Read the model definition and answer for the solid it produces. Units are mm, in the model's axes. Face numbers are marked on the shaded views. A direction names the side the tool comes from. Give positions to 0.01 mm unless a question says otherwise; leave off trailing zeros. Write each loop counter-clockwise with the first axis right and the second up, starting at its lowest first coordinate (ties: lowest second). Pieces come first, ordered by that corner, then holes. Notation, with made-up numbers: (-11.75, 57) -> (27.25, 57) arc R24 cw to (27.25, 78) -> close; hole circle Ø9 at (34.5, -11.5). An arc over 180 degrees is marked (long way). Answer as CSV lines item,"result". Start each with the question number.
1. Given pin 1 (1 mm diameter, centred on y = 27, z = 1, fed in from +X); pin 2 (19.5 mm diameter, centred on x = -9.5, z = -12.5, fed in from +Y); pin 3 (4.5 mm diameter, centred on x = -7.75, y = 12.78, fed in from -Z), each flat-ended and moving along its own axis, determine where each tip first touches the part or whether it passes through.
2. The part is cut by section B-B, the plane z = -27. Determine the outline of the cut face in (x, y), and give its area (3 significant figures).
3. The part is cut by section C-C, the plane x = -15. Determine the outline of the cut face in (y, z).
4. The part is cut by section A-A, the plane x = 0. Determine the outline of the cut face in (y, z).
5. The part is cut by section D-D, the plane x = 7.75. Determine the outline of the cut face in (y, z).
6. Find the intervals of material crossed by line 1 (Y direction, x = 7.75, z = 1.5); line 2 (Y direction, x = 7.75, z = 1.35); line 3 (Z direction, x = -9, y = 10.5), in increasing order.
7. A tool of negligible diameter and unlimited length cuts with its end or side. For the marked faces 1 and 2, from which of +Z, -Z, +X, -X, +Y, -Y can it reach the whole face along a straight path? Write none if from no direction.
from build123d import *

# Parameters (mm, degrees)
SKETCH_2_R          = 1.455943363
EXTRUDE_1_DEPTH     = 2
SKETCH_3_W          = 38.825156346
SKETCH_3_H          = 2
EXTRUDE_2_DEPTH     = 43
SKETCH_4_R          = 1.5
CUT_EXTRUDE_1_DEPTH = 10
FILLET_1_R          = 4
FILLET_2_R          = 2


with BuildPart() as part:
    # 草图2 → 凸台-拉伸1 (new body)
    with BuildSketch(Plane.XY):
        with BuildLine():
            Line((-19.412578173, 26.206980534), (-19.412578173, 0))
            Line((-19.412578173, 0), (19.412578173, 0))
            Line((19.412578173, 0), (19.412578173, 26.206980534))
            ThreePointArc((19.412578173, 26.206980534), (0, 45.619558707), (-19.412578173, 26.206980534))
        make_face()
        with Locations((15.5, 26.206980534)):
            Circle(SKETCH_2_R, mode=Mode.SUBTRACT)
        with Locations((7.75, 12.783586775)):
            Circle(SKETCH_2_R, mode=Mode.SUBTRACT)
        with Locations((-7.75, 12.783586775)):
            Circle(SKETCH_2_R, mode=Mode.SUBTRACT)
        with Locations((-15.5, 26.206980534)):
            Circle(SKETCH_2_R, mode=Mode.SUBTRACT)
        with Locations((-7.75, 39.630374293)):
            Circle(SKETCH_2_R, mode=Mode.SUBTRACT)
        with Locations((7.75, 39.630374293)):
            Circle(SKETCH_2_R, mode=Mode.SUBTRACT)
        with BuildLine():
            Line((-6.309087906, 33.206980534), (-6.309087906, 19.206980534))
            ThreePointArc((-6.309087906, 19.206980534), (0, 12.897892628), (6.309087906, 19.206980534))
            Line((6.309087906, 19.206980534), (6.309087906, 33.206980534))
            ThreePointArc((6.309087906, 33.206980534), (0, 39.51606844), (-6.309087906, 33.206980534))
        make_face(mode=Mode.SUBTRACT)
    extrude(amount=EXTRUDE_1_DEPTH)

    # 草图3 → 凸台-拉伸2 (add)
    with BuildSketch(Plane.XY.offset(2)):
        with Locations((0, 1)):
            Rectangle(SKETCH_3_W, SKETCH_3_H)
    extrude(amount=-EXTRUDE_2_DEPTH)

    # 草图4 → 切除-拉伸1 (cut)
    with BuildSketch(Plane(origin=(0, 2, 0), x_dir=(1, 0, 0), z_dir=(0, 1, 0))):
        with Locations(Location((-15, 7, 0), (0, 0, 270))):
            Circle(SKETCH_4_R)
        with Locations(Location((15, 7, 0), (0, 0, 270))):
            Circle(SKETCH_4_R)
        with BuildLine():
            Line((-16.5, 35), (-16.5, 25))
            ThreePointArc((-16.5, 25), (-15, 23.5), (-13.5, 25))
            Line((-13.5, 25), (-13.5, 35))
            ThreePointArc((-13.5, 35), (-15, 36.5), (-16.5, 35))
        make_face()
        with BuildLine():
            Line((13.5, 35), (13.5, 25))
            ThreePointArc((13.5, 25), (15, 23.5), (16.5, 25))
            Line((16.5, 25), (16.5, 35))
            ThreePointArc((16.5, 35), (15, 36.5), (13.5, 35))
        make_face()
    extrude(amount=-CUT_EXTRUDE_1_DEPTH, mode=Mode.SUBTRACT)

    # 圆角1
    fillet_1_edges = [part.edges().sort_by_distance(p)[0] for p in [
        (0, 0, 2),
    ]]
    fillet(fillet_1_edges, radius=FILLET_1_R)

    # 圆角2
    fillet_2_edges = [part.edges().sort_by_distance(p)[0] for p in [
        (0, 2, 0),
    ]]
    fillet(fillet_2_edges, radius=FILLET_2_R)


solid = part.part
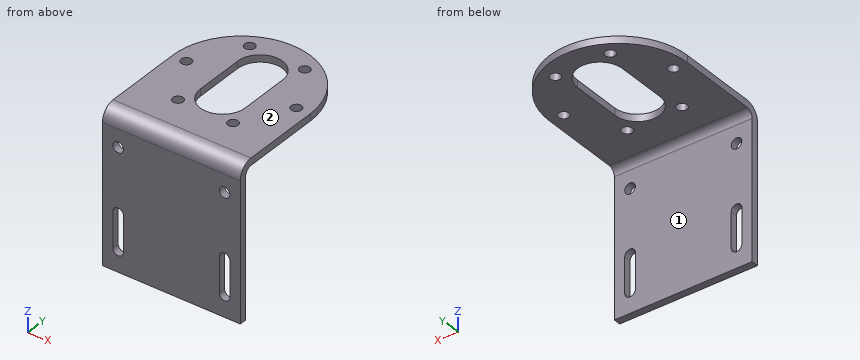
Results found:
1,pin 1,"stops at x = 19.41"
1,pin 2,"stops at y = 2"
1,pin 3,"stops at z = 0"
2,outline,"(-19.41, 0) -> (-16.5, 0) -> (-16.5, 2) -> (-19.41, 2) -> close; (-13.5, 0) -> (13.5, 0) -> (13.5, 2) -> (-13.5, 2) -> close; (16.5, 0) -> (19.41, 0) -> (19.41, 2) -> (16.5, 2) -> close"
2,area,"65.7 mm²"
3,outline,"(0, -41) -> (2, -41) -> (2, -36.5) -> (0, -36.5) -> close; (0, -23.5) -> (2, -23.5) -> (2, -8.5) -> (0, -8.5) -> close; (0, -5.5) -> (2, -5.5) -> (2, -2) arc R2 cw to (4, 0) -> (24.84, 0) -> (24.84, 2) -> (4, 2) arc R4 ccw to (0, -2) -> close; (27.57, 0) -> (38.53, 0) -> (38.53, 2) -> (27.57, 2) -> close"
4,outline,"(0, -41) -> (2, -41) -> (2, -2) arc R2 cw to (4, 0) -> (12.9, 0) -> (12.9, 2) -> (4, 2) arc R4 ccw to (0, -2) -> close; (39.52, 0) -> (45.62, 0) -> (45.62, 2) -> (39.52, 2) -> close"
5,outline,"(0, -41) -> (2, -41) -> (2, -2) arc R2 cw to (4, 0) -> (11.33, 0) -> (11.33, 2) -> (4, 2) arc R4 ccw to (0, -2) -> close; (14.24, 0) -> (38.17, 0) -> (38.17, 2) -> (14.24, 2) -> close; (41.09, 0) -> (44.01, 0) -> (44.01, 2) -> (41.09, 2) -> close"
6,line 1,"y = 2.06 to 11.33, 14.24 to 38.17, 41.09 to 44.01"
6,line 2,"y = 1.81 to 11.33, 14.24 to 38.17, 41.09 to 44.01"
6,line 3,"z = 0 to 2"
7,face 1,"-Z, +X, -X, +Y"
7,face 2,"+Z, +X, -X, +Y, -Y"
